Design review of the part built by this model. Coordinates are the model's own, in mm. Face numbers are marked on the shaded views. Round coordinates to 2 decimals unless told otherwise and drop trailing zeros. Use CSV: the item, a comma, the result in double quotes.
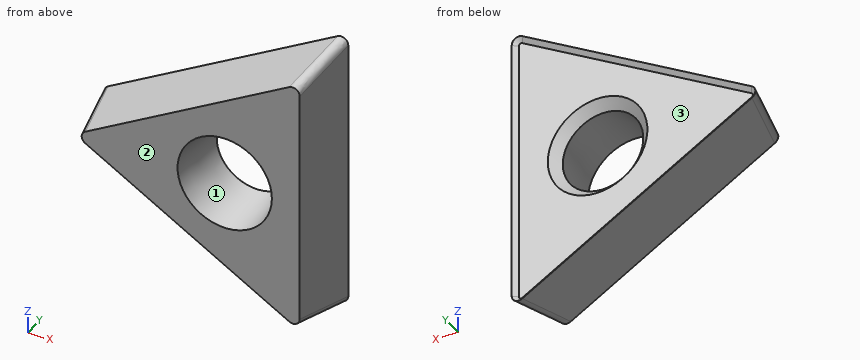
from build123d import *

# Parameters (mm, degrees)
F0_R     = 2.19964
F1_DEPTH = 3.97002
F1_TAPER = 7
F2_R     = 0.4064
F3_R     = 3.065431086
F4_DEPTH = 1.27
F4_TAPER = 45
F6_DEPTH = 0.2286
F6_TAPER = 50


# Not quite as in the source:
# - a feature names something its author has since deleted; it is built from what else it names


with BuildPart() as f1:
    # F0 (on Front) → F1 (new body)
    with BuildSketch(Plane.XZ):
        Polygon((4.7625, 8.248891971), (-9.525, 0), (4.7625, -8.248891971), align=None)
        Circle(F0_R, mode=Mode.SUBTRACT)
    extrude(amount=F1_DEPTH, taper=F1_TAPER)

    # F2
    f2_edges = [f1.edges().sort_by_distance(p)[0] for p in [
        (-9.037543, -1.98501, 0),
        (4.518771, -1.98501, 7.826742),
        (4.518771, -1.98501, -7.826742),
    ]]
    fillet(f2_edges, radius=F2_R)

    # F3 (on face) → F4 (cut)
    with BuildSketch(Plane.XZ):
        Circle(F3_R)
    extrude(amount=F4_DEPTH, taper=F4_TAPER, mode=Mode.SUBTRACT)

    # F5 (on face) → F6 (cut)
    with BuildSketch(Plane.XZ):
        with BuildLine():
            ThreePointArc((4.7625, 7.5449865229), (4.5593, 7.8969392469), (4.1529, 7.8969392469))
            Line((4.1529, 7.8969392469), (-8.9154, 0.3519527241))
            ThreePointArc((-8.9154, 0.3519527241), (-9.1186, 0), (-8.9154, -0.3519527241))
            Line((-8.9154, -0.3519527241), (4.1529, -7.8969392469))
            ThreePointArc((4.1529, -7.8969392469), (4.5593, -7.8969392469), (4.7625, -7.5449865229))
            Line((4.7625, -7.5449865229), (4.7625, 7.5449865229))
        make_face()
    extrude(amount=F6_DEPTH, taper=F6_TAPER, mode=Mode.SUBTRACT)


solid = f1.part
1) To check wall thickness, follow L1, parallel to Y at x = -3.5, z = 2.25; L2, parallel to X at y = -0.3, z = 1.5; L3, parallel to Z at x = -1.5, y = -1.3. State the ranges of each line that lie inside material, in increasing order. Write a range as from..to.
Data:
L1,"y = -3.97..-0.23"
L2,"x = -6.85..-2.32, 2.32..4.73"
L3,"z = -4.45..-1.82, 1.82..4.45"
2) The part is to be moulded in two halves that separate along X. For the marked faces 1, 2 and 3, say which applies: +X half, -X half, draft (parallel to the pull), parting line (faces both ways), or undercut.
Data:
face 1,"undercut"
face 2,"draft"
face 3,"undercut"
3) Insertion check: pin 1 Ø1 at (x, y) = (1, -2) entering from -Z. The pin has a flat end and moves straight along its axis. Give the tip position at first contact, or say it passes through.
Data:
pin 1,"stops at z = -6.09"
